Design review of the part built by this model. Coordinates are the model's own, in mm. A direction names the side the tool comes from. Round coordinates to 2 decimals unless told otherwise and drop trailing zeros. Loops run counter-clockwise (first coordinate to the right, second up) from the corner with the lowest first, then second, coordinate; pieces in that order, holes last. Notation, with made-up numbers: (-6.75, 31.5) - (48.25, 31.5) arc R6 cw to (48.25, 40.5) - close; hole circle Ø4 at (52.5, -15.75). An arc over 180 degrees is marked (long way). Return JSON: item names as keys, results as strings. Group by question number.
(1) We need section C-C, the plane x = 59. Write out the cut boundary in (y, z).
(2) Wall thickness on L1, parallel to Y at x = 47, z = 11.5; L2, parallel to Y at x = 59, z = -0.4; L3, parallel to X at y = 11, z = -0.6: over which ranges is each line inside the solid? List them lowest first. Write a range as [from, to].
(3) We need section D-D, the plane y = 13. Write out the cut boundary in (x, z).
(4) For faces 5 (the flat face through (58, 4, 4.5)), 6 (the flat face through (57, 1, -0.5)), 7 (the flat face through (57, 8, 1.5)), 8 (the flat face through (57.7, -13.5, 4)), 9 (the flat face through (57, 18, -0.5)), list the 3-axis set-ups (+Z, -Z, +X, -X, +Y, -Y) from which the entire face can be reached by the end or side of a thin tool; tool diameter is ignored.
(5) The part is to be moulded in two halves that separate along Y. For faces 1 (the flat face through (57, 7.1, -1)), 2 (the flat face through (47, 4, 20)), 3 (the cylindrical face through (47.5, -7.2, 13.1)), 4 (the flat face through (67.627, -12.655, 4.007)), say which applies: pulls with the +Y half, pulls with the -Y half, needs draft (parallel to the pull), parting line crosses it, or undercut.
(6) We need section B-B, the plane z = 11.5. Write out the cut boundary in (x, y).
(7) Clearance check with flat-ended pins moving along their axes: pin 1 (10.5 mm diameter, centred on x = 56, y = 13.5, fed in from +Z); pin 2 (4.5 mm diameter, centred on y = 7, z = 12, fed in from +X); pin 3 (1.5 mm diameter, centred on x = 53.5, z = 5, fed in from +Y). State where each tip first meets the part, or that it passes through.
(8) We need section A-A, the plane y = 3.5. Write out the cut boundary in (x, z), and give its area (3 significant figures).
from build123d import *

# Parameters (mm, degrees)
CYLINDER032_R         = 3.15
CYLINDER032_DEPTH     = 10
CYLINDER033_R         = 6.5
CYLINDER033_DEPTH     = 3
CYLINDER034_R         = 2.5
CYLINDER034_DEPTH     = 10
CYLINDER036_R         = 2
CYLINDER036_DEPTH     = 14
CYLINDER037_R         = 2
CYLINDER037_DEPTH     = 14
BOX059_W              = 3
BOX059_H              = 35
BOX059_DEPTH          = 20.5
FILLET005015029_R     = 3
CHAMFER010015007_SIZE = 0.4
BOX061_W              = 23
BOX061_H              = 9.5
BOX061_DEPTH          = 2
CHAMFER010015004_SIZE = 2
BOX062_W              = 23
BOX062_H              = 7.8
BOX062_DEPTH          = 1
BOX060_W              = 23
BOX060_H              = 35
BOX060_DEPTH          = 5
CHAMFER010015003_SIZE = 2
CHAMFER010015005_SIZE = 2
CHAMFER010015006_SIZE = 1
CHAMFER010015008_SIZE = 1


with BuildPart() as cylinder032:
    # Cylinder032 → Cylinder032 (new body)
    with BuildSketch(Plane(origin=(59, 11, -1.5), x_dir=(1, 0, 0), z_dir=(0, 0, 1))):
        Circle(CYLINDER032_R)
    extrude(amount=CYLINDER032_DEPTH)


with BuildPart() as fusion001021004009015013002:
    # Cylinder033 → Cylinder033 (new body)
    with BuildSketch(Plane(origin=(59, 11, 1.5), x_dir=(1, 0, 0), z_dir=(0, 0, 1))):
        Circle(CYLINDER033_R)
    extrude(amount=CYLINDER033_DEPTH)

    # Fusion001021004009015013002: union Cylinder032
    add(cylinder032.part)


with BuildPart() as cylinder034:
    # Cylinder034 → Cylinder034 (new body)
    with BuildSketch(Plane(origin=(42.5, 3.5, 11.5), x_dir=(0, 0, -1), z_dir=(1, 0, 0))):
        Circle(CYLINDER034_R)
    extrude(amount=CYLINDER034_DEPTH)


with BuildPart() as cylinder036:
    # Cylinder036 → Cylinder036 (new body)
    with BuildSketch(Plane(origin=(37, 13, 11.5), x_dir=(0, 0, -1), z_dir=(1, 0, 0))):
        Circle(CYLINDER036_R)
    extrude(amount=CYLINDER036_DEPTH)


with BuildPart() as fusion001021004009015013004:
    # Cylinder037 → Cylinder037 (new body)
    with BuildSketch(Plane(origin=(37, -6, 11.5), x_dir=(0, 0, -1), z_dir=(1, 0, 0))):
        Circle(CYLINDER037_R)
    extrude(amount=CYLINDER037_DEPTH)

    # Fusion001021004009015013004: union Cylinder034, Cylinder036
    add(cylinder034.part)
    add(cylinder036.part)


with BuildPart() as chamfer010015007:
    # Box059 → Box059 (new body)
    with BuildSketch(Plane(origin=(46, -14, -0.5), x_dir=(1, 0, 0), z_dir=(0, 0, 1))):
        with Locations((1.5, 17.5)):
            Rectangle(BOX059_W, BOX059_H)
    extrude(amount=BOX059_DEPTH)

    # Fillet005015029
    fillet005015029_edges = [chamfer010015007.edges().sort_by_distance(p)[0] for p in [
        (47.5, -14, 20),
        (47.5, 21, 20),
    ]]
    fillet(fillet005015029_edges, radius=FILLET005015029_R)

    # Chamfer010015007
    chamfer010015007_edges = [chamfer010015007.edges().sort_by_distance(p)[0] for p in [
        (49, -14, 8.25),
        (49, -13.12132, 19.12132),
        (49, 3.5, 20),
        (49, 21, 8.25),
        (49, 20.12132, 19.12132),
    ]]
    chamfer(chamfer010015007_edges, length=CHAMFER010015007_SIZE)


with BuildPart() as chamfer010015004:
    # Box061 → Box061 (new body)
    with BuildSketch(Plane(origin=(46, -14, -2.5), x_dir=(1, 0, 0), z_dir=(0, 0, 1))):
        with Locations((11.5, 4.75)):
            Rectangle(BOX061_W, BOX061_H)
    extrude(amount=BOX061_DEPTH)

    # Chamfer010015004
    chamfer010015004_edges = [chamfer010015004.edges().sort_by_distance(p)[0] for p in [
        (69, -14, -1.5),
    ]]
    chamfer(chamfer010015004_edges, length=CHAMFER010015004_SIZE)


with BuildPart() as cube060:
    # Box062 → Box062 (new body)
    with BuildSketch(Plane(origin=(46, 7.1, -1.5), x_dir=(1, 0, 0), z_dir=(0, 0, 1))):
        with Locations((11.5, 3.9)):
            Rectangle(BOX062_W, BOX062_H)
    extrude(amount=BOX062_DEPTH)


with BuildPart() as side_mount:
    # Box060 → Box060 (new body)
    with BuildSketch(Plane(origin=(46, -14, -0.5), x_dir=(1, 0, 0), z_dir=(0, 0, 1))):
        with Locations((11.5, 17.5)):
            Rectangle(BOX060_W, BOX060_H)
    extrude(amount=BOX060_DEPTH)

    # Chamfer010015003
    chamfer010015003_edges = [side_mount.edges().sort_by_distance(p)[0] for p in [
        (69, -14, 2),
    ]]
    chamfer(chamfer010015003_edges, length=CHAMFER010015003_SIZE)

    # Chamfer010015005
    chamfer010015005_edges = [side_mount.edges().sort_by_distance(p)[0] for p in [
        (69, 21, 2),
    ]]
    chamfer(chamfer010015005_edges, length=CHAMFER010015005_SIZE)

    # Chamfer010015006
    chamfer010015006_edges = [side_mount.edges().sort_by_distance(p)[0] for p in [
        (69, 3.5, 4.5),
        (68, 20, 4.5),
        (56.5, 21, 4.5),
        (56.5, -14, 4.5),
        (68, -13, 4.5),
    ]]
    chamfer(chamfer010015006_edges, length=CHAMFER010015006_SIZE)

    # Fusion001021004009015013005: union Chamfer010015007, Chamfer010015004, Cube060
    add(chamfer010015007.part)
    add(chamfer010015004.part)
    add(cube060.part)

    # Cut019003009: cut Fusion001021004009015013004
    add(fusion001021004009015013004.part, mode=Mode.SUBTRACT)

    # Chamfer010015008
    chamfer010015008_edges = [side_mount.edges().sort_by_distance(p)[0] for p in [
        (49, 3.5, 14),
    ]]
    chamfer(chamfer010015008_edges, length=CHAMFER010015008_SIZE)

    # Cut019003010: cut Fusion001021004009015013002
    add(fusion001021004009015013002.part, mode=Mode.SUBTRACT)


solid = side_mount.part
Solutions:
{
 "1": {"outline": "(-14, -2.5) - (-4.5, -2.5) - (-4.5, -0.5) - (7.1, -0.5) - (7.1, -1.5) - (7.85, -1.5) - (7.85, 1.5) - (4.5, 1.5) - (4.5, 4.5) - (-13, 4.5) - (-14, 3.5) - close; (14.15, -1.5) - (14.9, -1.5) - (14.9, -0.5) - (21, -0.5) - (21, 3.5) - (20, 4.5) - (17.5, 4.5) - (17.5, 1.5) - (14.15, 1.5) - close"},
 "2": {"L1": "[-14, -8], [-4, 1], [6, 11], [15, 21]", "L2": "[-14, 7.85], [14.15, 21]", "L3": "[46, 55.85], [62.15, 69]"},
 "3": {"outline": "(46, -1.5) - (56.57, -1.5) - (56.57, 1.5) - (52.82, 1.5) - (52.82, 4.5) - (49, 4.5) - (49, 9.5) - (46, 9.5) - close; (46, 13.5) - (49, 13.5) - (49, 19.6) - (48.6, 20) - (46, 20) - close; (61.43, -1.5) - (69, -1.5) - (69, 3.5) - (68, 4.5) - (65.18, 4.5) - (65.18, 1.5) - (61.43, 1.5) - close"},
 "4": {"face 5": "+Z, +X, +Y, -Y", "face 6": "-Z, +X, -X", "face 7": "+Z", "face 8": "+Z, +X, -Y", "face 9": "-Z, +X, -X, +Y"},
 "5": {"face 1": "undercut", "face 2": "needs draft", "face 3": "undercut", "face 4": "pulls with the -Y half"},
 "6": {"outline": "(46, -14) - (48.6, -14) - (49, -13.6) - (49, -8) - (46, -8) - close; (46, -4) - (49, -4) - (49, 0) - (48, 1) - (46, 1) - close; (46, 6) - (48, 6) - (49, 7) - (49, 11) - (46, 11) - close; (46, 15) - (49, 15) - (49, 20.6) - (48.6, 21) - (46, 21) - close"},
 "7": {"pin 1": "z = 4.5", "pin 2": "x = 49", "pin 3": "y = 20.25"},
 "8": {"outline": "(46, -0.5) - (69, -0.5) - (69, 3.5) - (68, 4.5) - (49, 4.5) - (49, 8) - (48, 9) - (46, 9) - close; (46, 14) - (48, 14) - (49, 15) - (49, 19.6) - (48.6, 20) - (46, 20) - close", "area": "145 mm^2"}
}
